Could you check a few things on this model? Use its own coordinates, in mm. A direction names the side the tool comes from. Give positions to 0.01 mm unless a question says otherwise; leave off trailing zeros. Order: outer loops, then holes, each group sorted by start corner. A loop starts at its lowest first (then second) coordinate and runs counter-clockwise, first axis right, second up. Notation, with made-up numbers: (22, 83) -> (33, 83) arc R17 cw to (33, 93) -> close; hole circle Ø2 at (76, -30). An arc over 180 degrees is marked (long way). One line per item, written item: value.
Autodesk Inventor part; units mm, degrees
ref_plane "YZ Plane" through (0, 0, 0) normal (1, 0, 0) x (0, 1, 0)
ref_plane "XZ Plane" through (0, 0, 0) normal (0, 1, 0) x (-1, 0, 0)
ref_plane "XY Plane" through (0, 0, 0) normal (0, 0, 1) x (1, 0, 0)
ref_plane "Work Plane1" through (0, 0, 0) normal (0, 0, 1) x (1, 0, 0)
sketch "Sketch1" plane through (0, 0, 0) normal (0, 0, 1) x (1, 0, 0)
  arc A0 (-148.6847, 77.7603) -> (-148.1357, 75.7112) centre (-147.3857, 77.0103) ccw
  line L0 (-148.6847, 77.7603) -> (-148.1847, 78.6263)
  line L1 (-148.1847, 78.6263) -> (-150.7828, 80.1263)
  line L2 (-150.7828, 80.1263) -> (-152.7828, 76.6622)
  arc A1 (-155.3809, 78.1622) -> (-152.7828, 76.6622) centre (-154.0818, 77.4122) ccw
  line L3 (-155.3809, 78.1622) -> (-158.3253, 79.8622)
  arc A2 (-156.8253, 82.4603) -> (-158.3253, 79.8622) centre (-157.5753, 81.1612) ccw
  line L4 (-156.8253, 82.4603) -> (-156.3253, 83.3263)
  line L5 (-156.3253, 83.3263) -> (-161.1751, 86.1263)
  arc A3 (-159.9251, 88.2913) -> (-161.1751, 86.1263) centre (-160.5501, 87.2088) ccw
  line L6 (-159.9251, 88.2913) -> (-155.0753, 85.4913)
  line L7 (-155.0753, 85.4913) -> (-151.5753, 91.5535)
  line L8 (-151.5753, 91.5535) -> (-156.4251, 94.3535)
  arc A4 (-155.1751, 96.5186) -> (-156.4251, 94.3535) centre (-155.8001, 95.4361) ccw
  line L9 (-155.1751, 96.5186) -> (-150.3253, 93.7186)
  line L10 (-150.3253, 93.7186) -> (-149.8253, 94.5846)
  arc A5 (-148.3253, 97.1827) -> (-149.8253, 94.5846) centre (-149.0753, 95.8836) ccw
  line L11 (-148.3253, 97.1827) -> (-145.3809, 95.4827)
  arc A6 (-142.7828, 93.9827) -> (-145.3809, 95.4827) centre (-144.0818, 94.7327) ccw
  line L12 (-142.7828, 93.9827) -> (-144.7828, 90.5186)
  line L13 (-144.7828, 90.5186) -> (-142.1847, 89.0186)
  line L14 (-142.1847, 89.0186) -> (-141.6847, 89.8846)
  arc A7 (-139.6357, 90.4336) -> (-141.6847, 89.8846) centre (-140.3857, 89.1346) ccw
  line L15 (-139.6357, 90.4336) -> (-134.9591, 87.7336)
  arc A8 (-134.4101, 85.6846) -> (-134.9591, 87.7336) centre (-135.7091, 86.4346) ccw
  line L16 (-134.4101, 85.6846) -> (-136.9101, 81.3545)
  line L17 (-136.9101, 81.3545) -> (-133.7924, 79.5545)
  arc A9 (-135.7924, 76.0904) -> (-133.7924, 79.5545) centre (-134.7924, 77.8224) ccw
  line L18 (-135.7924, 76.0904) -> (-138.9101, 77.8904)
  line L19 (-138.9101, 77.8904) -> (-141.4101, 73.5603)
  arc A10 (-143.4591, 73.0112) -> (-141.4101, 73.5603) centre (-142.7091, 74.3103) ccw
  line L20 (-143.4591, 73.0112) -> (-148.1357, 75.7112)
  arc A11 (141.6847, 89.8846) -> (139.6357, 90.4336) centre (140.3857, 89.1346) ccw
  line L21 (141.6847, 89.8846) -> (142.1847, 89.0186)
  line L22 (142.1847, 89.0186) -> (144.7828, 90.5186)
  line L23 (144.7828, 90.5186) -> (142.7828, 93.9827)
  arc A12 (145.3809, 95.4827) -> (142.7828, 93.9827) centre (144.0818, 94.7327) ccw
  line L24 (145.3809, 95.4827) -> (148.3253, 97.1827)
  arc A13 (149.8253, 94.5846) -> (148.3253, 97.1827) centre (149.0753, 95.8836) ccw
  line L25 (149.8253, 94.5846) -> (150.3253, 93.7186)
  line L26 (150.3253, 93.7186) -> (155.1751, 96.5186)
  arc A14 (156.4251, 94.3535) -> (155.1751, 96.5186) centre (155.8001, 95.4361) ccw
  line L27 (156.4251, 94.3535) -> (151.5753, 91.5535)
  line L28 (151.5753, 91.5535) -> (155.0753, 85.4913)
  line L29 (155.0753, 85.4913) -> (159.9251, 88.2913)
  arc A15 (161.1751, 86.1263) -> (159.9251, 88.2913) centre (160.5501, 87.2088) ccw
  line L30 (161.1751, 86.1263) -> (156.3253, 83.3263)
  line L31 (156.3253, 83.3263) -> (156.8253, 82.4603)
  arc A16 (158.3253, 79.8622) -> (156.8253, 82.4603) centre (157.5753, 81.1612) ccw
  line L32 (158.3253, 79.8622) -> (155.3809, 78.1622)
  arc A17 (152.7828, 76.6622) -> (155.3809, 78.1622) centre (154.0818, 77.4122) ccw
  line L33 (152.7828, 76.6622) -> (150.7828, 80.1263)
  line L34 (150.7828, 80.1263) -> (148.1847, 78.6263)
  line L35 (148.1847, 78.6263) -> (148.6847, 77.7603)
  arc A18 (148.1357, 75.7112) -> (148.6847, 77.7603) centre (147.3857, 77.0103) ccw
  line L36 (148.1357, 75.7112) -> (143.4591, 73.0112)
  arc A19 (141.4101, 73.5603) -> (143.4591, 73.0112) centre (142.7091, 74.3103) ccw
  line L37 (141.4101, 73.5603) -> (138.9101, 77.8904)
  line L38 (138.9101, 77.8904) -> (135.7924, 76.0904)
  arc A20 (133.7924, 79.5545) -> (135.7924, 76.0904) centre (134.7924, 77.8224) ccw
  line L39 (133.7924, 79.5545) -> (136.9101, 81.3545)
  line L40 (136.9101, 81.3545) -> (134.4101, 85.6846)
  arc A21 (134.9591, 87.7336) -> (134.4101, 85.6846) centre (135.7091, 86.4346) ccw
  line L41 (134.9591, 87.7336) -> (139.6357, 90.4336)
  line L42 (6, -167.6449) -> (6, -170.6449)
  line L43 (6, -170.6449) -> (10, -170.6449)
  arc A22 (10, -173.6449) -> (10, -170.6449) centre (10, -172.1449) ccw
  line L44 (10, -173.6449) -> (10, -177.0449)
  arc A23 (7, -177.0449) -> (10, -177.0449) centre (8.5, -177.0449) ccw
  line L45 (7, -177.0449) -> (6, -177.0449)
  line L46 (6, -177.0449) -> (6, -182.6449)
  arc A24 (3.5, -182.6449) -> (6, -182.6449) centre (4.75, -182.6449) ccw
  line L47 (3.5, -182.6449) -> (3.5, -177.0449)
  line L48 (3.5, -177.0449) -> (-3.5, -177.0449)
  line L49 (-3.5, -177.0449) -> (-3.5, -182.6449)
  arc A25 (-6, -182.6449) -> (-3.5, -182.6449) centre (-4.75, -182.6449) ccw
  line L50 (-6, -182.6449) -> (-6, -177.0449)
  line L51 (-6, -177.0449) -> (-7, -177.0449)
  arc A26 (-10, -177.0449) -> (-7, -177.0449) centre (-8.5, -177.0449) ccw
  line L52 (-10, -177.0449) -> (-10, -173.6449)
  arc A27 (-10, -170.6449) -> (-10, -173.6449) centre (-10, -172.1449) ccw
  line L53 (-10, -170.6449) -> (-6, -170.6449)
  line L54 (-6, -170.6449) -> (-6, -167.6449)
  line L55 (-6, -167.6449) -> (-7, -167.6449)
  arc A28 (-8.5, -166.1449) -> (-7, -167.6449) centre (-7, -166.1449) ccw
  line L56 (-8.5, -166.1449) -> (-8.5, -160.7449)
  arc A29 (-7, -159.2449) -> (-8.5, -160.7449) centre (-7, -160.7449) ccw
  line L57 (-7, -159.2449) -> (-2, -159.2449)
  line L58 (-2, -159.2449) -> (-2, -155.6449)
  arc A30 (2, -155.6449) -> (-2, -155.6449) centre (0, -155.6449) ccw
  line L59 (2, -155.6449) -> (2, -159.2449)
  line L60 (2, -159.2449) -> (7, -159.2449)
  arc A31 (8.5, -160.7449) -> (7, -159.2449) centre (7, -160.7449) ccw
  line L61 (8.5, -160.7449) -> (8.5, -166.1449)
  arc A32 (7, -167.6449) -> (8.5, -166.1449) centre (7, -166.1449) ccw
  line L62 (7, -167.6449) -> (6, -167.6449)
  arc A33 (174.3732, -22.7321) -> (67.5, 162.3777) centre (67.5, 38.9711) ccw
  line L63 (67.5, 162.3777) -> (-67.5, 162.3777)
  arc A34 (-67.5, 162.3777) -> (-174.3732, -22.7321) centre (-67.5, 38.9711) ccw
  line L64 (-174.3732, -22.7321) -> (-106.8732, -139.6455)
  arc A35 (-106.8732, -139.6455) -> (106.8732, -139.6455) centre (0, -77.9423) ccw
  line L65 (106.8732, -139.6455) -> (174.3732, -22.7321)
  circle A36 centre (160.7436, 60.4737) radius 2
  circle A37 centre (132.7436, 108.9711) radius 2
  circle A38 centre (-160.7436, 60.4737) radius 2
  circle A39 centre (-132.7436, 108.9711) radius 2
  circle A40 centre (28, -169.4449) radius 2
  circle A41 centre (-28, -169.4449) radius 2
  circle A42 centre (0, 0) radius 5
  circle A43 centre (-28, -169.4449) radius 7
  circle A44 centre (28, -169.4449) radius 7
  line L66 (-12, -155.6449) -> (12, -155.6449)
  line L67 (12, -155.6449) -> (12, -185.6449)
  line L68 (12, -185.6449) -> (-12, -185.6449)
  line L69 (-12, -185.6449) -> (-12, -155.6449)
  line L70 (-30.5576, -162.9288) -> (-12, -155.6449)
  line L71 (-31.227, -175.6567) -> (-12, -185.6449)
  line L72 (31.227, -175.6567) -> (12, -185.6449)
  line L73 (30.5576, -162.9288) -> (12, -155.6449)
  line L74 (-7, -159.2449) -> (7, -159.2449)
  line L75 (8.5, -160.7449) -> (8.5, -166.1449)
  line L76 (7, -167.6449) -> (-7, -167.6449)
  line L77 (-8.5, -166.1449) -> (-8.5, -160.7449)
  line L78 (-10, -170.6449) -> (10, -170.6449)
  line L79 (10, -170.6449) -> (10, -177.0449)
  line L80 (10, -177.0449) -> (-10, -177.0449)
  line L81 (-10, -177.0449) -> (-10, -170.6449)
  arc A45 (-7, -159.2449) -> (-8.5, -160.7449) centre (-7, -160.7449) ccw
  arc A46 (-8.5, -166.1449) -> (-7, -167.6449) centre (-7, -166.1449) ccw
  arc A47 (7, -167.6449) -> (8.5, -166.1449) centre (7, -166.1449) ccw
  arc A48 (8.5, -160.7449) -> (7, -159.2449) centre (7, -160.7449) ccw
  circle A49 centre (-28, -169.4449) radius 2.15
  circle A50 centre (28, -169.4449) radius 2.15
  point P0 (0, 0)
  dimension "d2" = 14
  dimension "d3" = 14
  dimension "d5" = 30
  dimension "d6" = 2
  dimension "d7" = 2
  dimension "d8" = 1.5
  dimension "d16" = 4.3
  dimension "d17" = 4.3
extrude "Extrusion1" add sketch "Sketch1" along normal blind 1.5 contours L62 A32 L61 A31 L60 L59 L66 L67 L68 L69 L58 L57 A29 L56 A28 L55 L54 L53 A27 L52 A26 L51 L50 A25 L49 L48 L47 A24 L46 L45 A23 L44 A22 L43 L42 | L42 L78 L54 L76 | A22 L79 | L81 A27 | A23 L80 | L80 A26 | L74 L58 L66 L59 | L46 A24 L47 L80 | L80 L49 A25 L50 | L73 A44 L72 L67 | L69 L71 A43 L70 | A44 | A43
fillet "Fillet1" radius 30 4 edges at (-12, -185.6449, 0.75) (12, -185.6449, 0.75) (-12, -155.6449, 0.75) (12, -155.6449, 0.75)
sketch "Sketch2" plane through (0, 0, 1.5) normal (0, 0, 1) x (1, 0, 0)
  line L0 (10, -177.0449) -> (-10, -177.0449)
  circle A0 centre (0, -182.0449) radius 1.5
  point P0 (0, 0)
  dimension "d12" = 3
  dimension "d13" = 5
extrude "Extrusion2" cut sketch "Sketch2" against normal blind 10
properties material "Stainless Steel"
1) For P1, Ø0.8, axis at y = -163, z = 0.5, coming from the -X side, with a flat end and sliding along its axis, tell me the tip position at first contact or that it passes through.
Answer below:
P1: stops at x = -31.53
2) Suppose I cut it at D-D, the plane z = 0.85. Write out the boundary of the cut face in (x, y).
Answer below:
outline: (-31.23, -175.66) -> (-18.5, -182.27) arc R30 ccw to (-4.67, -185.64) -> (4.67, -185.64) arc R30 ccw to (18.5, -182.27) -> (31.23, -175.66) arc R7 ccw to (30.56, -162.93) -> (17.28, -157.72) arc R30 ccw to (6.32, -155.64) -> (-6.32, -155.64) arc R30 ccw to (-17.28, -157.72) -> (-30.56, -162.93) arc R7 ccw to start; hole circle Ø4.3 at (-28, -169.44); hole (-10, -177.04) -> (10, -177.04) -> (10, -170.64) -> (-10, -170.64) -> close; hole (-8.5, -166.14) arc R1.5 ccw to (-7, -167.64) -> (7, -167.64) arc R1.5 ccw to (8.5, -166.14) -> (8.5, -160.74) arc R1.5 ccw to (7, -159.24) -> (-7, -159.24) arc R1.5 ccw to (-8.5, -160.74) -> close; hole circle Ø3 at (0, -182.04); hole circle Ø4.3 at (28, -169.44)
3) Suppose I cut it at B-B, the plane x = -28. Write out the boundary of the cut face in (y, z), then the cut area to 3 significant figures.
Answer below:
outline: (-177.33, 0) -> (-171.59, 0) -> (-171.59, 1.5) -> (-177.33, 1.5) -> close; (-167.29, 0) -> (-161.92, 0) -> (-161.92, 1.5) -> (-167.29, 1.5) -> close
area: 16.7 mm2
4) If I drill on line 1 along Y through (x, z) = (0, 0.5); line 2 along Y through (x, z) = (-5, 0.3); line 3 along X through (y, z) = (-168.25, 0.45), over which ranges is the centre line in solid material (lowest first)?
Answer below:
line 1: y = -185.64 to -183.54, -180.54 to -177.04, -170.64 to -167.64, -159.24 to -155.64
line 2: y = -185.64 to -177.04, -170.64 to -167.64, -159.24 to -155.64
line 3: x = -34.9 to -29.79, -26.21 to 26.21, 29.79 to 34.9
5) For faces 4 (the cylindrical face through (11.978, -156.183, 0.76)), 5 (the flat face through (0, -177.045, 1)), which set-ups out of +Z, -Z, +X, -X, +Y, -Y let a thin tool reach every point of the face, with its end or its side?
Answer below:
face 4: +Z, -Z, +X, +Y
face 5: +Z, -Z
6) Suppose I cut it at A-A, the plane x = 0. Write out the boundary of the cut face in (y, z).
Answer below:
outline: (-185.64, 0) -> (-183.54, 0) -> (-183.54, 1.5) -> (-185.64, 1.5) -> close; (-180.54, 0) -> (-177.04, 0) -> (-177.04, 1.5) -> (-180.54, 1.5) -> close; (-170.64, 0) -> (-167.64, 0) -> (-167.64, 1.5) -> (-170.64, 1.5) -> close; (-159.24, 0) -> (-155.64, 0) -> (-155.64, 1.5) -> (-159.24, 1.5) -> close
7) Suppose I cut it at C-C, the plane y = -160. Write out the boundary of the cut face in (x, z), then the cut area to 3 significant figures.
Answer below:
outline: (-23.1, 0) -> (-8.3, 0) -> (-8.3, 1.5) -> (-23.1, 1.5) -> close; (8.3, 0) -> (23.1, 0) -> (23.1, 1.5) -> (8.3, 1.5) -> close
area: 44.4 mm2
8) We'd pull the mould along X, two halves only. Please class faces 1 (the flat face through (0, -185.645, 1)), 2 (the cylindrical face through (-0.33, -183.51, 0.76)), 3 (the cylindrical face through (34.984, -168.965, 0.74)): +X half, -X half, draft (parallel to the pull), parting line (faces both ways), or undercut.
Answer below:
face 1: draft
face 2: undercut
face 3: +X half
